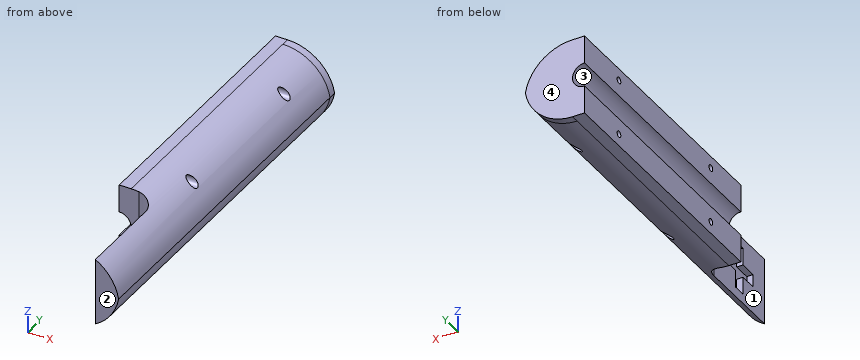
from build123d import *

# Parameters (mm, degrees)
BOSS_EXTRU_1_DEPTH            = 50
CONG_4_R                      = 35
CONG_5_R                      = 35
CONG_6_R                      = 30
CONG_12_R                     = 10
ENL_V_MAT_EXTRU_8_DEPTH       = 251
ESQUISSE6_R                   = 2
ENL_V_MAT_EXTRU_9_DEPTH       = 58
ENL_V_MAT_EXTRU_12_DEPTH      = 251.898527225
ENL_V_MAT_EXTRU_12_DEPTH_BACK = 179
ESQUISSE11_R                  = 3
ENL_V_MAT_EXTRU_14_DEPTH      = 20
BOSS_EXTRU_2_DEPTH            = 5
ESQUISSE13_W                  = 8
ESQUISSE13_H                  = 30
ESQUISSE13_W_2                = 30
ESQUISSE13_H_2                = 8
ENL_V_MAT_EXTRU_15_DEPTH      = 4


with BuildPart() as part:
    # Esquisse1 → Boss.-Extru.1 (new body)
    with BuildSketch(Plane.XY):
        Polygon((-129.391143911, 131.10701107), (-129.391143911, -98.89298893), (-124.391143911, -98.89298893), (-124.391143911, -33.89298893), (-64.391143911, -33.89298893), (-64.391143911, -98.89298893), (-49.391143911, -98.89298893), (-49.391143911, 131.10701107), align=None)
    extrude(amount=BOSS_EXTRU_1_DEPTH)

    # Congé4
    cong_4_edges = [part.edges().sort_by_distance(p)[0] for p in [
        (-129.391143911, 16.10701107, 50),
    ]]
    fillet(cong_4_edges, radius=CONG_4_R)

    # Congé5
    # the kernel refuses this fillet: 35 mm, written as the material it takes off along each edge
    with BuildSketch(Plane(origin=(-129.391143911, 202.914044152, 0), x_dir=(0, 0, 1), z_dir=(0, -1, 0))) as cong_5_piece_1:
        with BuildLine():
            CenterArc((35, -28.722813233), CONG_5_R, 124.849904579, 55.150095421)
            Line((0, -28.722813233), (-0.7, -28.722813233))
            Line((-0.7, -28.722813233), (-0.7, 0))
            Line((-0.7, 0), (0, 0.7))
            ThreePointArc((0, 0.7), (7.5, 0.7), (14.6, 0.574456265))
            Line((14.6, 0.574456265), (15, 0))
        make_face()
    extrude(amount=373.614066163, mode=Mode.SUBTRACT)

    # Congé6
    # the kernel refuses this fillet: 30 mm, written as the material it takes off along each edge
    with BuildSketch(Plane(origin=(-49.391143911, -173.89298893, 0), x_dir=(-1, 0, 0), z_dir=(0, 1, 0))) as cong_6_piece_1:
        with BuildLine():
            CenterArc((CONG_6_R, CONG_6_R), CONG_6_R, 180, 90)
            Line((0, CONG_6_R), (0, 0))
            Line((0, 0), (CONG_6_R, 0))
        make_face()
    extrude(amount=380, mode=Mode.SUBTRACT)
    with BuildSketch(Plane(origin=(-49.391143911, -173.89298893, 50), x_dir=(-1, 0, 0), z_dir=(0, 1, 0))) as cong_6_piece_2:
        with BuildLine():
            CenterArc((CONG_6_R, -CONG_6_R), CONG_6_R, 90, 90)
            Line((0, -CONG_6_R), (0, 0))
            Line((0, 0), (CONG_6_R, 0))
        make_face()
    extrude(amount=380, mode=Mode.SUBTRACT)

    # Congé12
    cong_12_edges = [part.edges().sort_by_distance(p)[0] for p in [
        (-124.391143911, -33.89298893, 21.146981396),
        (-64.391143911, -33.89298893, 25),
    ]]
    fillet(cong_12_edges, radius=CONG_12_R)

    # Esquisse5 → Enlèv. mat.-Extru.8 (cut)
    with BuildSketch(Plane(origin=(0, 131.10701107, 0), x_dir=(1, 0, 0), z_dir=(0, 1, 0))):
        with BuildLine():
            Line((-86.891143911, -50), (-86.891143911, 0))
            ThreePointArc((-86.891143911, 0), (-162.141280076, -25), (-86.891143911, -50))
        make_face()
    extrude(amount=-ENL_V_MAT_EXTRU_8_DEPTH, mode=Mode.SUBTRACT)

    # Esquisse6 → Enlèv. mat.-Extru.9 (cut)
    with BuildSketch(Plane.ZY.offset(86.891143911)):
        with Locations((7.5, 98.60701107)):
            Circle(ESQUISSE6_R)
        with Locations((42.5, 98.60701107)):
            Circle(ESQUISSE6_R)
        with Locations((42.5, -1.39298893)):
            Circle(ESQUISSE6_R)
        with Locations((7.5, -1.39298893)):
            Circle(ESQUISSE6_R)
    extrude(amount=-ENL_V_MAT_EXTRU_9_DEPTH, mode=Mode.SUBTRACT)

    # Esquisse9 → Enlèv. mat.-Extru.12 (cut, two sides: drawn at the far end of the back side and taken through both)
    with BuildSketch(Plane(origin=(0, 131.10701107, 0), x_dir=(1, 0, 0), z_dir=(0, 1, 0)).offset(-ENL_V_MAT_EXTRU_12_DEPTH_BACK)):
        with BuildLine():
            Line((-195.505666121, -17.5), (-86.891143911, -17.5))
            ThreePointArc((-86.891143911, -17.5), (-79.391143911, -25), (-86.891143911, -32.5))
            Line((-86.891143911, -32.5), (-195.505666121, -32.5))
            Line((-195.505666121, -32.5), (-412.73471054, -32.5))
            Line((-412.73471054, -32.5), (-412.73471054, -17.5))
            Line((-412.73471054, -17.5), (-195.505666121, -17.5))
        make_face()
    extrude(amount=ENL_V_MAT_EXTRU_12_DEPTH + ENL_V_MAT_EXTRU_12_DEPTH_BACK, mode=Mode.SUBTRACT)

    # Esquisse11 → Enlèv. mat.-Extru.14 (cut)
    with BuildSketch(Plane.ZY.offset(49.810744996)):
        with Locations(Location((42.5, 98.60701107, 0), (0, 0, 180))):
            Circle(ESQUISSE11_R)
        with Locations(Location((7.5, 98.60701107, 0), (0, 0, 180))):
            Circle(ESQUISSE11_R)
        with Locations(Location((42.5, -1.39298893, 0), (0, 0, 180))):
            Circle(ESQUISSE11_R)
        with Locations(Location((7.5, -1.39298893, 0), (0, 0, 180))):
            Circle(ESQUISSE11_R)
    extrude(amount=ENL_V_MAT_EXTRU_14_DEPTH, mode=Mode.SUBTRACT)

    # Esquisse12 → Boss.-Extru.2 (add)
    with BuildSketch(Plane(origin=(0, 131.10701107, 0), x_dir=(1, 0, 0), z_dir=(0, 1, 0))):
        with BuildLine():
            Line((-79.391143911, 0), (-86.891143911, 0))
            Line((-86.891143911, 0), (-86.891143911, -17.5))
            ThreePointArc((-86.891143911, -17.5), (-79.391143911, -25), (-86.891143911, -32.5))
            Line((-86.891143911, -32.5), (-86.891143911, -50))
            Line((-86.891143911, -50), (-79.391143911, -50))
            ThreePointArc((-79.391143911, -50), (-60.02622718, -42.912878475), (-49.810744996, -25))
            ThreePointArc((-49.810744996, -25), (-60.02622718, -7.087121525), (-79.391143911, 0))
        make_face()
    extrude(amount=BOSS_EXTRU_2_DEPTH)

    # Esquisse13 → Enlèv. mat.-Extru.15 (cut)
    with BuildSketch(Plane.ZY.offset(64.391143911)):
        with Locations((25, -71.39298893)):
            Rectangle(ESQUISSE13_W, ESQUISSE13_H)
        with Locations((25, -71.39298893)):
            Rectangle(ESQUISSE13_W_2, ESQUISSE13_H_2)
    extrude(amount=-ENL_V_MAT_EXTRU_15_DEPTH, mode=Mode.SUBTRACT)


solid = part.part
Geometry: final body of the model. Coordinates: model frame, mm. Face numbers are marked on the shaded views. A direction names the side the tool comes from. Give positions to 0.01 mm unless a question says otherwise; leave off trailing zeros. Loops run counter-clockwise (first coordinate to the right, second up) from the corner with the lowest first, then second, coordinate; pieces in that order, holes last. Notation, with made-up numbers: M -39.75,34 L -8.75,34 A21 ccw -8.75,48 Z; hole C 48.5,64 d11. An arc over 180 degrees is marked long. Put each result on its own line as item: value.
1) Cut plane A-A, the plane y = 36. Return the cut outline in (x, z).
Computed values:
outline: M -86.89,0 L -79.39,0 A30 ccw -49.81,25 A30 ccw -79.39,50 L -86.89,50 L -86.89,32.5 A7.5 cw -86.89,17.5 Z
2) Material intervals for L1, parallel to Y at x = -60.25, z = 42.5; L2, parallel to Y at x = -66.25, z = 42.5; L3, parallel to Y at x = -61.5, z = 25, sorted ascending. Write a range as from..to.
Computed values:
L1: y = -98.89..-4.39, 1.61..95.61, 101.61..136.11
L2: y = -38.09..-4.39, 1.61..95.61, 101.61..136.11
L3: y = -98.89..-86.39, -56.39..136.11
3) Cut plane C-C, the plane x = -54. Return the cut outline in (y, z).
Computed values:
outline: M -98.89,14.02 L 136.11,14.02 L 136.11,35.98 L -98.89,35.98 Z
4) First-contact query: P1, Ø10, axis at x = -73.5, z = 8, coming from the -Y side; P2, Ø12, axis at x = -63.5, y = 56, coming from the +Z side; P3, Ø5, axis at y = 98.61, z = 42.5, coming from the +X side; P4, Ø8, axis at y = -1.39, z = 42.5, coming from the -X side. Flat tips, straight axial feed; report the tip coordinate or a pass-through.
Computed values:
P1: stops at y = -35.81
P2: stops at z = 48.32
P3: stops at x = -69.81
P4: stops at x = -86.89
5) Mould query, pull axis Z, two halves, no side actions, for the marked faces 3 and 4. Classes: released by +Z, released by -Z, zero draft, split by the parting line, or undercut.
Computed values:
face 3: undercut
face 4: zero draft
6) Reachability of the marked faces 1 and 2 from +Z, -Z, +X, -X, +Y, -Y: full face, straight path, thin tool, end or side. Return the list, or none.
Computed values:
face 1: +Z, -Z, -X, -Y
face 2: +Z, -Z, +X, -X, -Y
7) Cut plane B-B, the plane z = 7.5. Return the cut outline in (x, y).
Computed values:
outline: M -86.89,-33.89 L -74.39,-33.89 A10 cw -64.39,-43.89 L -64.39,-98.89 L -59.55,-98.89 L -59.55,-4.39 L -69.81,-4.39 L -69.81,-3.39 L -86.89,-3.39 Z; M -86.89,0.61 L -69.81,0.61 L -69.81,1.61 L -59.55,1.61 L -59.55,95.61 L -69.81,95.61 L -69.81,96.61 L -86.89,96.61 Z; M -86.89,100.61 L -69.81,100.61 L -69.81,101.61 L -59.55,101.61 L -59.55,136.11 L -86.89,136.11 Z
